Autodesk Inventor part; units mm, degrees
ref_plane "YZ Plane" through (0, 0, 0) normal (1, 0, 0) x (0, 1, 0)
ref_plane "XZ Plane" through (0, 0, 0) normal (0, 1, 0) x (-1, 0, 0)
ref_plane "XY Plane" through (0, 0, 0) normal (0, 0, 1) x (1, 0, 0)
sketch "Sketch1" plane through (0, 0, 0) normal (0, 0, 1) x (1, 0, 0)
  circle A0 centre (0, 0) radius 0.9779
  dimension "d0" = 1.9558
extrude "Extrusion1" add sketch "Sketch1" against normal blind 2.6162
sketch "Sketch2" plane through (0, 0, -2.6162) normal (0, 0, -1) x (-1, 0, 0)
  circle A0 centre (0, 0) radius 1.7272
  dimension "d3" = 3.4544
extrude "Extrusion2" add sketch "Sketch2" along normal blind 0.9652
sketch "Sketch3" plane through (0, 0, -3.5814) normal (0, 0, -1) x (-1, 0, 0)
  circle A0 centre (0, 0) radius 0.9779
extrude "Extrusion3" add sketch "Sketch3" along normal blind 7.7724
sketch "Sketch4" plane through (0, 0, -11.3538) normal (0, 0, -1) x (-1, 0, 0)
  circle A0 centre (0, 0) radius 8.001
  dimension "d8" = 16.002
extrude "Extrusion4" add sketch "Sketch4" along normal blind 0.8382
sketch "Sketch5" plane through (0, 0, -12.192) normal (0, 0, -1) x (-1, 0, 0)
  circle A0 centre (0, 0) radius 8.001
  circle A1 centre (0, 0) radius 2.5146
  point P0 (-4.9792, 6.2629)
  point P1 (-3.3536, 7.2643)
  point P2 (-1.728, 7.8122)
  point P3 (-0.1024, 8.0003)
  point P4 (1.5232, 7.8547)
  point P5 (5.0214, 6.2291)
  point P6 (6.544, 4.6035)
  point P7 (7.4262, 2.9779)
  point P8 (7.8859, 1.3523)
  point P9 (7.9963, -0.2733)
  point P10 (7.7724, -1.8989)
  point P11 (7.1829, -3.5245)
  point P12 (6.1231, -5.1501)
  point P13 (4.4975, -6.6173)
  point P14 (2.8719, -7.4678)
  point P15 (1.2463, -7.9033)
  point P16 (-0.3793, -7.992)
  point P17 (-2.0049, -7.7457)
  point P18 (-3.6305, -7.1299)
  point P19 (-5.2561, -6.0323)
  point P20 (-6.8817, -4.0814)
  point P21 (-7.6148, -2.4558)
  point P22 (-7.9578, -0.8302)
  point P23 (-7.9614, 0.7954)
  point P24 (-7.6259, 2.421)
  point P25 (-6.9023, 4.0466)
  point P26 (-5.6429, 5.6722)
  point P27 (-3.3816, 7.2513)
  dimension "d11" = 1.6256
  dimension "d12" = 1.6256
  dimension "d13" = 1.6256
  dimension "d14" = 1.6256
  dimension "d15" = 1.6256
  dimension "d16" = 1.6256
  dimension "d17" = 1.6256
  dimension "d18" = 1.6256
  dimension "d19" = 1.6256
  dimension "d20" = 1.6256
  dimension "d21" = 1.6256
  dimension "d22" = 1.6256
  dimension "d23" = 1.6256
  dimension "d24" = 1.6256
  dimension "d25" = 1.6256
  dimension "d26" = 1.6256
  dimension "d27" = 1.6256
  dimension "d28" = 1.6256
  dimension "d29" = 1.6256
  dimension "d30" = 1.6256
  dimension "d32" = 1.6256
  dimension "d33" = 1.6256
  dimension "d34" = 1.6256
  dimension "d35" = 1.6256
  dimension "d36" = 1.6256
  dimension "d37" = 1.6256
  dimension "d39" = 5.0292
extrude "Extrusion5" add sketch "Sketch5" along normal blind 2.8448 contours A1
sketch "Sketch6" plane through (0, 0, -15.0368) normal (0, 0, -1) x (-1, 0, 0)
  circle A0 centre (0, 0) radius 0.9779
  dimension "d42" = 1.9558
extrude "Extrusion6" add sketch "Sketch6" along normal blind 2.4892
sketch "Sketch8" plane through (0, 0, -12.192) normal (0, 0, -1) x (-1, 0, 0)
  point P0 (0, 0)
sketch "Sketch9" plane through (0, 0, -12.192) normal (0, 0, -1) x (-1, 0, 0)
  circle A0 centre (0, 0) radius 8.001
  circle A1 centre (0, 0) radius 9.6774
  line L0 (0, 8.001) -> (0.9393, 9.6317)
  line L1 (0.9393, 9.6317) -> (1.5623, 7.847)
  line L2 (1.5623, 7.847) -> (2.7497, 9.2785)
  line L3 (2.7497, 9.2785) -> (3.0623, 7.3918)
  line L4 (3.0623, 7.3918) -> (4.4462, 8.5955)
  line L5 (4.4462, 6.6518) -> (5.9473, 7.6343)
  line L6 (5.9473, 7.6343) -> (5.6517, 5.6634)
  line L7 (5.6517, 5.6634) -> (7.4382, 6.1907)
  line L8 (7.4382, 6.1907) -> (6.494, 4.6738)
  line L9 (6.494, 4.6738) -> (8.4739, 4.6738)
  line L10 (8.4739, 4.6738) -> (7.2714, 3.3381)
  line L11 (7.2714, 3.3381) -> (9.2449, 2.8608)
  line L12 (9.2449, 2.8608) -> (7.7959, 1.8)
  line L13 (7.7959, 1.8) -> (9.6193, 1.0592)
  line L14 (9.6193, 1.0592) -> (8.001, 0)
  line L15 (8.001, 0) -> (9.6193, -1.0592)
  line L16 (9.6193, -1.0592) -> (7.7959, -1.8)
  line L17 (7.7959, -1.8) -> (9.2096, -2.9725)
  line L18 (7.2714, -3.3381) -> (9.2096, -2.9725)
  line L19 (7.2714, -3.3381) -> (8.4739, -4.6738)
  line L20 (8.4739, -4.6738) -> (6.494, -4.6738)
  line L21 (6.494, -4.6738) -> (7.4212, -6.2111)
  line L22 (7.4212, -6.2111) -> (5.6517, -5.6634)
  line L23 (5.6517, -5.6634) -> (6.253, -7.3859)
  line L24 (6.253, -7.3859) -> (4.4462, -6.6518)
  line L25 (4.4462, -6.6518) -> (4.4462, -8.5955)
  line L26 (4.4462, -8.5955) -> (3.0623, -7.3918)
  line L27 (3.0623, -7.3918) -> (2.7497, -9.2785)
  line L28 (2.7497, -9.2785) -> (1.5623, -7.847)
  line L29 (1.5623, -7.847) -> (1.0123, -9.6243)
  line L30 (1.0123, -9.6243) -> (0, -8.001)
  line L31 (0, -8.001) -> (-1.0386, -9.6215)
  line L32 (-1.0386, -9.6215) -> (-1.5623, -7.847)
  line L33 (-1.5623, -7.847) -> (-2.9628, -9.2127)
  line L34 (-2.9628, -9.2127) -> (-3.0623, -7.3918)
  line L35 (-3.0623, -7.3918) -> (-4.7392, -8.4375)
  line L36 (-4.4437, -6.6536) -> (-4.7392, -8.4375)
  line L37 (-4.4437, -6.6536) -> (-6.2508, -7.3878)
  line L38 (-6.2508, -7.3878) -> (-5.6517, -5.6634)
  line L39 (-5.6517, -5.6634) -> (-7.6188, -5.967)
  line L40 (-7.6188, -5.967) -> (-6.494, -4.6738)
  line L41 (-6.494, -4.6738) -> (-8.5183, -4.5924)
  line L42 (-8.5183, -4.5924) -> (-7.2714, -3.3381)
  line L43 (-7.2714, -3.3381) -> (-9.2096, -2.9725)
  line L44 (-9.2096, -2.9725) -> (-7.7959, -1.8)
  line L45 (-7.7959, -1.8) -> (-9.6399, -0.851)
  line L46 (-9.6399, -0.851) -> (-8.001, 0)
  line L47 (-8.001, 0) -> (-9.612, 1.1235)
  line L48 (-9.612, 1.1235) -> (-7.7959, 1.8)
  line L49 (-7.7959, 1.8) -> (-9.1513, 3.1474)
  line L50 (-9.1513, 3.1474) -> (-7.2714, 3.3381)
  line L51 (-8.4739, 4.6738) -> (-7.2714, 3.3381)
  line L52 (-8.4739, 4.6738) -> (-6.494, 4.6738)
  line L53 (-6.494, 4.6738) -> (-7.3128, 6.3383)
  line L54 (-7.3128, 6.3383) -> (-5.6517, 5.6634)
  line L55 (-5.6517, 5.6634) -> (-6.1785, 7.4483)
  line L56 (-6.1785, 7.4483) -> (-4.4437, 6.6536)
  line L57 (-4.4437, 6.6536) -> (-4.4437, 8.5969)
  line L58 (-4.4437, 8.5969) -> (-3.0595, 7.3929)
  line L59 (-3.0595, 7.3929) -> (-2.6348, 9.3118)
  line L60 (-2.6348, 9.3118) -> (-1.5623, 7.847)
  line L61 (-1.5623, 7.847) -> (-0.9432, 9.6313)
  line L62 (0, 8.001) -> (-0.9432, 9.6313)
  line L63 (4.4462, 6.6518) -> (4.4462, 8.5955)
  point P0 (-4.4462, 6.6518)
  dimension "d71" = 19.3548
extrude "Extrusion7" add sketch "Sketch9" against normal blind 0.8382 contours L15 L16 A0 | A0 L13 L14 | A0 L11 L12 | L17 L18 A0 | A0 L9 L10 | L19 L20 A0 | A0 L7 L8 | L21 L22 A0 | A0 L5 L6 | L23 L24 A0 | A0 L4 L63 | L25 L26 A0 | A0 L2 L3 | L27 L28 A0 | A0 L0 L1 | L29 L30 A0 | A0 L61 L62 | L31 L32 A0 | A0 L59 L60 | L33 L34 A0 | A0 L57 L58 | L35 L36 A0 | A0 L55 L56 | L37 L38 A0 | A0 L53 L54 | L39 L40 A0 | A0 L51 L52 | L41 L42 A0 | A0 L49 L50 | L43 L44 A0 | A0 L47 L48 | L45 L46 A0
properties part number "gear" material "Aluminum 6061"
Can you work these out from the model? Positions are in its coordinate system, mm. A direction names the side the tool comes from. Round coordinates to 2 decimals unless told otherwise and drop trailing zeros. Loops run counter-clockwise (first coordinate to the right, second up) from the corner with the lowest first, then second, coordinate; pieces in that order, holes last. Notation, with made-up numbers: (59.25, -29) -> (75.25, -29) arc R7 cw to (75.25, -25) -> close; hole circle Ø1 at (86.25, -10). An arc over 180 degrees is marked (long way). One line per item, written item: value. Start each with the question number.
1. For pin 1 (0.9 mm diameter, centred on y = -7.5, z = -12, fed in from -X); pin 2 (3 mm diameter, centred on x = -2, y = 6.5, fed in from -Z); pin 3 (0.9 mm diameter, centred on y = 7.5, z = -12, fed in from +X), each with a flat end and sliding along its axis, tell me the tip position at first contact or that it passes through.
2. If we section it at A-A, the plane y = 7: Write out the boundary of the cut face in (x, z), then the cut area to 3 significant figures.
3. If we mould it in two halves opening along X, with no side actions, what happens to faces 6 (the flat face through (-6.55, -5.94, -11.78)), 7 (the flat face through (-7.864, -3.997, -11.779)), 8 (the cylindrical face through (0.933, 0.294, -1.29))? For each: pulls with the +X half, pulls with the -X half, needs draft (parallel to the pull), parting line crosses it, or undercut.
4. If we section it at C-C, the plane y = -3.75: Write out the boundary of the cut face in (x, z).
5. If we section it at B-B, the plane z = -8: Write out the boundary of the cut face in (x, y).
6. If I drill on probe 1 along Z at (x, y) = (3, 2); probe 2 along Y at (x, z) = (-0.25, -15); probe 3 along X at (y, z) = (-5.5, -11.5), over which ranges is the centre line in solid material (lowest first)?
7. For faces 1 (the flat face through (7.881, 4.015, -11.779)), 2 (the flat face through (-2.16, -8.57, -11.78)), 3 (the flat face through (5.3, -7, -11.8)), 4 (the flat face through (-4.446, 8, -12)), 5 (the flat face through (-8.821, 0.537, -11.779)), which set-ups out of +Z, -Z, +X, -X, +Y, -Y let a thin tool reach every point of the face, with its end or its side?
Calculated:
1. pin 1: stops at x = -6.25
1. pin 2: stops at z = -12.19
1. pin 3: stops at x = 6.18
2. outline: (-5.85, -12.19) -> (-4.98, -12.19) -> (-4.98, -11.35) -> (-5.85, -11.35) -> close; (-4.45, -12.19) -> (4.44, -12.19) -> (4.44, -11.35) -> (-4.45, -11.35) -> close; (5.2, -12.19) -> (6.05, -12.19) -> (6.05, -11.35) -> (5.2, -11.35) -> close
2. area: 8.89 mm²
3. face 6: undercut
3. face 7: pulls with the -X half
3. face 8: parting line crosses it
4. outline: (-7.64, -12.19) -> (7.68, -12.19) -> (7.68, -11.35) -> (-7.64, -11.35) -> close
5. outline: circle Ø1.96 at (0, 0)
6. probe 1: z = -12.19 to -11.35
6. probe 2: y = -2.5 to 2.5
6. probe 3: x = -6.99 to 7.21
7. face 1: +Z, -Z, +X
7. face 2: +Z, -Z, -Y
7. face 3: +Z, -Z
7. face 4: +Z, -Z, +Y
7. face 5: +Z, -Z, -X
